Check sheet for the drawn part. Datum: minimum x, y, z corner. Units: mm. A direction names the side the tool comes from. Give positions to 0.01 mm unless a question says otherwise; leave off trailing zeros. Write each loop counter-clockwise with the first axis right and the second up, starting at its lowest first coordinate (ties: lowest second). Pieces come first, ordered by that corner, then holes. Notation, with made-up numbers: (69.5, 3) -> (76.5, 3) arc R19 cw to (76.5, 24) -> close; hole circle Ø6 at (71, 43.5). An arc over 180 degrees is marked (long way). Use CSV: the item, a comma, the result in double quotes. Start each with the question number.
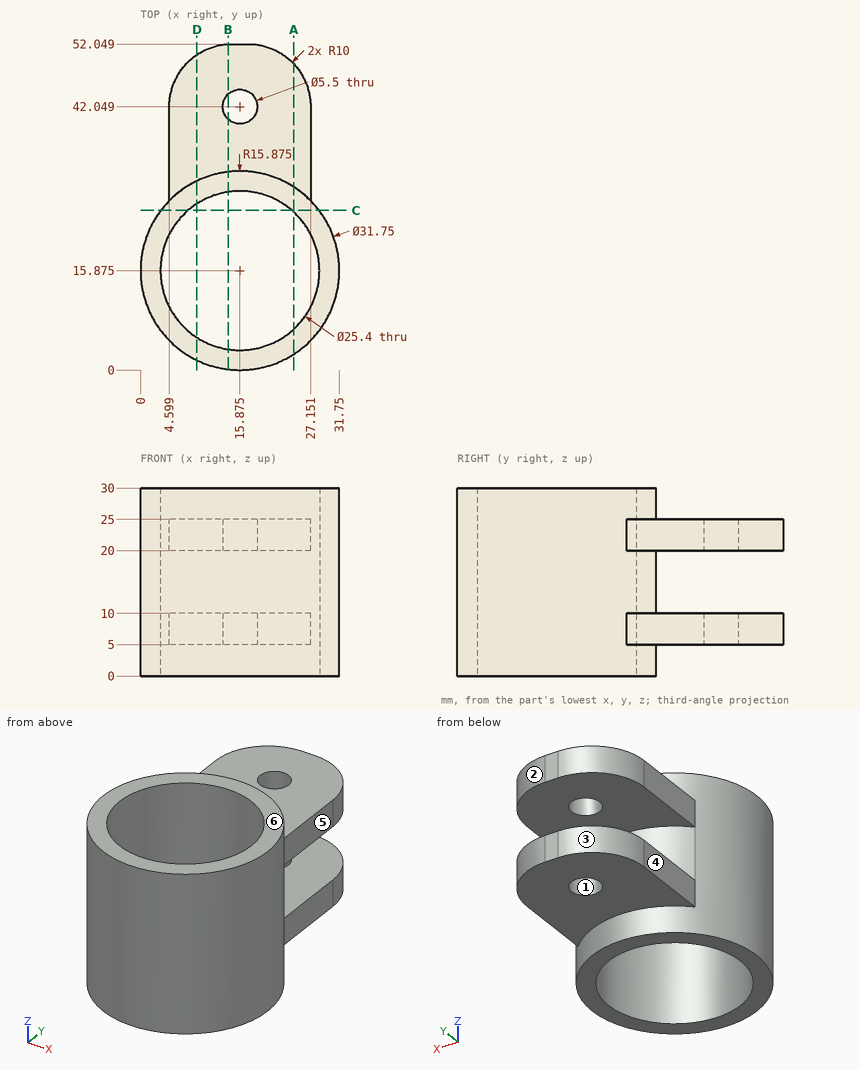
(1) Set-up check for the marked faces 4, 5 and 6: record each of +Z, -Z, +X, -X, +Y, -Y from which the full face is reachable in a straight line by a thin tool's end or side.
(2) Go/stop test with flat-tipped pins: pin 1 (7 mm diameter, centred on x = 15.88, y = 42.05, fed in from +Z); pin 2 (2.5 mm diameter, centred on y = 35, z = 8, fed in from +X); pin 3 (1 mm diameter, centred on x = 12, z = 21.5, fed in from -Y). Record where each tip stops, or that it passes through.
(3) Section check D-D on x = 9. Record the cut outline in (y, z) (1 decimal).
(4) Section check A-A on x = 24.5. Record the cut outline in (y, z).
(5) Section check B-B on x = 14. Record the cut outline in (y, z).
(6) Section check C-C on y = 25.5. Record the cut outline in (x, z), then the cut area to 3 significant figures.
(7) Thickness scan on line 1 (Z direction, x = 12, y = 38.5); line 2 (Y direction, x = 8.5, z = 15.5) (1 decimal); line 3 (X direction, y = 13, z = 24.25) (1 decimal). Record the ranges inside material, lowest first. Write a range as from..to.
(8) Draft check along X on the marked faces 1, 2 and 3. Enter one of: released by +X, released by -X, zero draft, split by the parting line, or undercut.
Data:
1,face 4,"+Z, -Z, -X, +Y"
1,face 5,"+Z, -Z, +X, +Y"
1,face 6,"+Z, +X, -X, +Y, -Y"
2,pin 1,"stops at z = 25"
2,pin 2,"stops at x = 27.15"
2,pin 3,"stops at y = 0.36"
3,outline,"(1.6, 0) -> (5.2, 0) -> (5.2, 30) -> (1.6, 30) -> close; (26.6, 0) -> (30.2, 0) -> (30.2, 5) -> (50.3, 5) -> (50.3, 10) -> (30.2, 10) -> (30.2, 20) -> (50.3, 20) -> (50.3, 25) -> (30.2, 25) -> (30.2, 30) -> (26.6, 30) -> close"
4,outline,"(2.55, 0) -> (6.55, 0) -> (6.55, 30) -> (2.55, 30) -> close; (25.2, 0) -> (29.2, 0) -> (29.2, 5) -> (48.83, 5) -> (48.83, 10) -> (29.2, 10) -> (29.2, 20) -> (48.83, 20) -> (48.83, 25) -> (29.2, 25) -> (29.2, 30) -> (25.2, 30) -> close"
5,outline,"(0.11, 0) -> (3.31, 0) -> (3.31, 30) -> (0.11, 30) -> close; (28.44, 0) -> (31.64, 0) -> (31.64, 5) -> (40.04, 5) -> (40.04, 10) -> (31.64, 10) -> (31.64, 20) -> (40.04, 20) -> (40.04, 25) -> (31.64, 25) -> (31.64, 30) -> (28.44, 30) -> close; (44.06, 5) -> (52.03, 5) -> (52.03, 10) -> (44.06, 10) -> close; (44.06, 20) -> (52.03, 20) -> (52.03, 25) -> (44.06, 25) -> close"
6,outline,"(3.25, 0) -> (7.59, 0) -> (7.59, 30) -> (3.25, 30) -> close; (24.16, 0) -> (28.5, 0) -> (28.5, 30) -> (24.16, 30) -> close"
6,area,"260 mm2"
7,line 1,"z = 5..10, 20..25"
7,line 2,"y = 1.8..5.5, 26.2..29.9"
7,line 3,"x = 0.3..3.5, 28.2..31.5"
8,face 1,"undercut"
8,face 2,"released by +X"
8,face 3,"released by -X"
